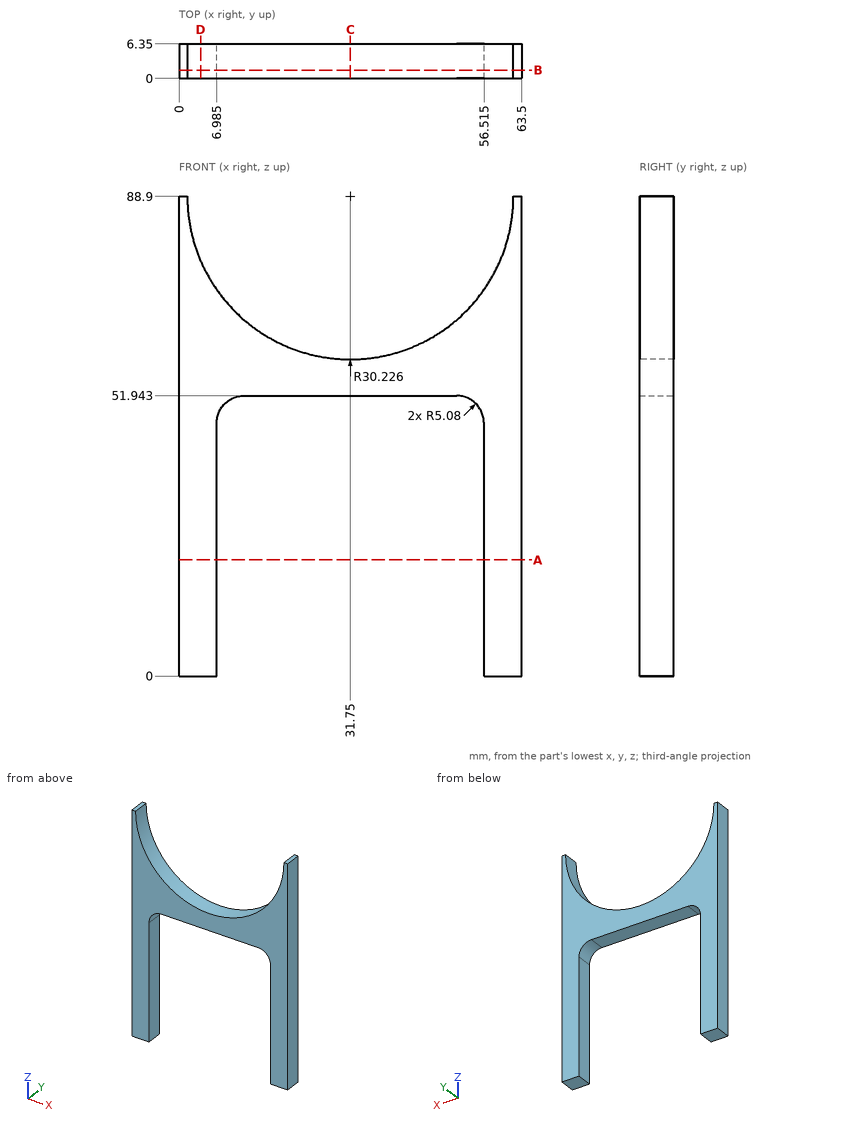
Part print with two shaded views. Sizes in mm from the minimum x, y, z corner. Round coordinates to 2 decimals unless told otherwise and drop trailing zeros. Loops run counter-clockwise (first coordinate to the right, second up) from the corner with the lowest first, then second, coordinate; pieces in that order, holes last. Notation, with made-up numbers: (64, -25.5) - (94, -25.5) arc R8 cw to (94, -19.5) - close; hole circle Ø2 at (74, 67.25). An arc over 180 degrees is marked (long way). Put each result on its own line as item: value.
1. Slice it at D-D on x = 4. List the corners of the cut face in (y, z), and give its area (3 significant figures).
Geometry check:
outline: (0, 0) - (6.35, 0) - (6.35, 76.92) - (0, 76.92) - close
area: 488 mm²
2. Pin check, flat tips, straight feed: P1, Ø3, axis at x = 16.5, y = 5, coming from the -Z side; P2, Ø1, axis at x = 9.5, y = 0.5, coming from the +Z side; P3, Ø3, axis at x = 11, y = 5.5, coming from the +Z side. Stop position of each tip, or through.
Geometry check:
P1: z = 51.94
P2: z = 69
P3: z = 68.44
3. Slice it at B-B on y = 1.5. List the corners of the cut face in (x, z) (3 decimals), and give its area (3 significant figures).
Geometry check:
outline: (0, 0) - (6.985, 0) - (6.985, 46.863) arc R5.08 cw to (12.065, 51.943) - (51.435, 51.943) arc R5.08 cw to (56.515, 46.863) - (56.515, 0) - (63.5, 0) - (63.5, 88.9) - (61.976, 88.9) arc R30.226 cw to (1.524, 88.9) - (0, 88.9) - close
area: 1,650 mm²
4. Wall check: line 1 (X direction, y = 3, z = 16.5) (3 decimals); line 2 (X direction, y = 0.75, z = 82); line 3 (Z direction, x = 17, y = 4.5). Give the ranges that are in metal, low to high.
Geometry check:
line 1: 0 to 6.985, 56.515 to 63.5
line 2: 0 to 2.32, 61.18 to 63.5
line 3: 51.94 to 62.52
5. Slice it at A-A on z = 21.5. List the corners of the cut face in (x, y) (3 decimals), and give its area (3 significant figures).
Geometry check:
outline: (0, 0) - (6.985, 0) - (6.985, 6.35) - (0, 6.35) - close; (56.515, 0) - (63.5, 0) - (63.5, 6.35) - (56.515, 6.35) - close
area: 88.7 mm²
6. Slice it at C-C on x = 31.75. List the corners of the cut face in (y, z), and give its area (3 significant figures).
Geometry check:
outline: (0, 51.94) - (6.35, 51.94) - (6.35, 58.67) - (0, 58.67) - close
area: 42.7 mm²
